Check sheet for the modelled part. Datum: model origin and axes. Units: mm. A direction names the side the tool comes from. Round coordinates to 2 decimals unless told otherwise and drop trailing zeros. Order: outer loops, then holes, each group sorted by start corner. A loop starts at its lowest first (then second) coordinate and runs counter-clockwise, first axis right, second up.
(1) Tool access check on faces 4 (the cylindrical face through (12.25, -9.51, 1.5)), 5 (the cylindrical face through (0.39, -0.6, 6.93)). Record the directions out of +Z, -Z, +X, -X, +Y, -Y that give a thin tool (end or side, any length) a straight path to the whole face; none if there is none.
(2) Thickness scan on probe 1 along Z at (x, y) = (-18.5, -10); probe 2 along Y at (x, z) = (-23.5, -4.25); probe 3 along X at (y, z) = (-0.5, -3.5). Record the ranges inside material, lowest first.
(3) Sectioned sample at C-C, the plane x = -24. Enter the section's corners in (y, z).
(4) Depth check by flat-ended pin: pin 1 (8 mm diameter, centred on x = 9.5, z = 1.5, fed in from -Y); pin 2 (9 mm diameter, centred on x = 22.48, z = 0, fed in from -Y); pin 3 (1 mm diameter, centred on x = 19.5, y = -1, fed in from -Z). Enter the tip coordinate at first touch or a pass-through.
(5) Sectioned sample at B-B, the plane z = 0. Enter the section's corners in (x, y), and give its area (3 significant figures).
(6) Sectioned sample at D-D, the plane z = -2.5. Enter the section's corners in (x, y).
(7) Mould release check, pull along Z, two halves, no side actions. Record for faces 1 (the flat face through (30, -5, 0)), 2 (the cylindrical face through (27.25, -9.51, 1.5)), 3 (the cylindrical face through (0.39, -9.9, -6.93)): released by +Z, released by -Z, zero draft, split by the parting line, or undercut.
(8) Sectioned sample at A-A, the plane x = -15.5. Enter the section's corners in (y, z), and give its area (3 significant figures).
```python
from build123d import *

# Parameters (mm, degrees)
F0_W     = 60
F0_H     = 15
F1_DEPTH = 10.5
F2_R     = 5
F3_DEPTH = 2
F4_R     = 2


# Not quite as in the source:
# - a feature names something its author has since deleted; it is built from what else it names


with BuildPart() as f1:
    # F0 (on Front) → F1 (new body)
    with BuildSketch(Plane.XZ):
        Rectangle(F0_W, F0_H)
    extrude(amount=F1_DEPTH)

    # F2 (on face) → F3 (cut)
    with BuildSketch(Plane.XZ.offset(10.5)):
        with Locations((-22.5179158151, 0)):
            Circle(F2_R)
        with Locations((-7.5179158151, 0)):
            Circle(F2_R)
        with Locations((7.4820841849, 0)):
            Circle(F2_R)
        with Locations((22.4820841849, 0)):
            Circle(F2_R)
    extrude(amount=-F3_DEPTH, mode=Mode.SUBTRACT)

    # F4
    f4_edges = [f1.edges().sort_by_distance(p)[0] for p in [
        (-30, -5.25, 7.5),
        (30, 0, 0),
        (0, -10.5, 7.5),
        (0, 0, 7.5),
        (30, -5.25, 7.5),
        (30, -5.25, -7.5),
        (30, -10.5, 0),
        (0, 0, -7.5),
        (-30, 0, 0),
        (-30, -5.25, -7.5),
        (-30, -10.5, 0),
        (0, -10.5, -7.5),
    ]]
    fillet(f4_edges, radius=F4_R)


solid = f1.part
```
Derived:
1. face 4: -Y
1. face 5: +Z, +X, -X, +Y
2. probe 1: z = -6.82 to -2.98, 2.98 to 6.82
2. probe 2: y = -8.5 to 0
2. probe 3: x = -29.32 to 29.32
3. outline: (-10.5, -5.5) arc R2 ccw to (-8.5, -7.5) - (-2, -7.5) arc R2 ccw to (0, -5.5) - (0, 5.5) arc R2 ccw to (-2, 7.5) - (-8.5, 7.5) arc R2 ccw to (-10.5, 5.5) - (-10.5, 4.78) - (-8.5, 4.78) - (-8.5, -4.78) - (-10.5, -4.78) - close
4. pin 1: stops at y = -10.5
4. pin 2: stops at y = -8.5
4. pin 3: stops at z = -7.44
5. outline: (-30, -8.5) arc R2 ccw to (-28, -10.5) - (-27.52, -10.5) - (-27.52, -8.5) - (-17.52, -8.5) - (-17.52, -10.5) - (-12.52, -10.5) - (-12.52, -8.5) - (-2.52, -8.5) - (-2.52, -10.5) - (2.48, -10.5) - (2.48, -8.5) - (12.48, -8.5) - (12.48, -10.5) - (17.48, -10.5) - (17.48, -8.5) - (27.48, -8.5) - (27.48, -10.5) - (28, -10.5) arc R2 ccw to (30, -8.5) - (30, -2) arc R2 ccw to (28, 0) - (-28, 0) arc R2 ccw to (-30, -2) - close
5. area: 547 mm2
6. outline: (-30, -8.5) arc R2 ccw to (-28, -10.5) - (-26.85, -10.5) - (-26.85, -8.5) - (-18.19, -8.5) - (-18.19, -10.5) - (-11.85, -10.5) - (-11.85, -8.5) - (-3.19, -8.5) - (-3.19, -10.5) - (3.15, -10.5) - (3.15, -8.5) - (11.81, -8.5) - (11.81, -10.5) - (18.15, -10.5) - (18.15, -8.5) - (26.81, -8.5) - (26.81, -10.5) - (28, -10.5) arc R2 ccw to (30, -8.5) - (30, -2) arc R2 ccw to (28, 0) - (-28, 0) arc R2 ccw to (-30, -2) - close
7. face 1: zero draft
7. face 2: undercut
7. face 3: released by -Z
8. outline: (-10.5, -5.5) arc R2 ccw to (-8.5, -7.5) - (-2, -7.5) arc R2 ccw to (0, -5.5) - (0, 5.5) arc R2 ccw to (-2, 7.5) - (-8.5, 7.5) arc R2 ccw to (-10.5, 5.5) - close
8. area: 154 mm2
